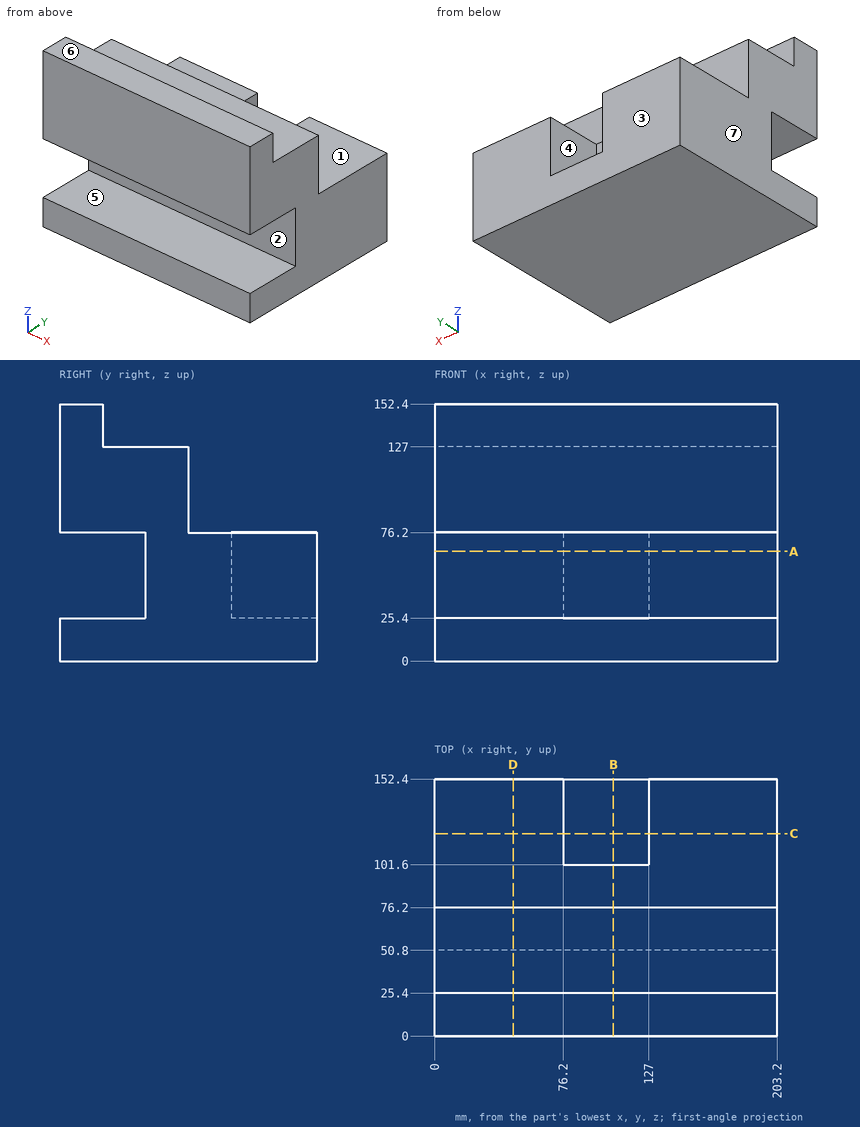
Print and shaded views of the part. All mm, measured from the part's lowest x, y and z. A direction names the side the tool comes from. Round coordinates to 2 decimals unless told otherwise and drop trailing zeros. Loops run counter-clockwise (first coordinate to the right, second up) from the corner with the lowest first, then second, coordinate; pieces in that order, holes last. Notation, with made-up numbers: M -19.75,-5.75 L 9.25,-5.75 A26 ccw 9.25,22.25 Z; hole C 80,26 d8. An arc over 180 degrees is marked long. One line per question, with ' | ' between items.
1) Band-saw the part on A-A (z = 65). Give the cut face in (x, y), then the cut area to 3 significant figures.
Solved:
outline: M 0,50.8 L 203.2,50.8 L 203.2,152.4 L 127,152.4 L 127,101.6 L 76.2,101.6 L 76.2,152.4 L 0,152.4 Z | area: 18,100 mm²
2) Band-saw the part on D-D (x = 46.5). Give the cut face in (y, z).
Solved:
outline: M 0,0 L 152.4,0 L 152.4,76.2 L 76.2,76.2 L 76.2,127 L 25.4,127 L 25.4,152.4 L 0,152.4 L 0,76.2 L 50.8,76.2 L 50.8,25.4 L 0,25.4 Z
3) Band-saw the part on C-C (y = 120). Give the cut face in (x, z).
Solved:
outline: M 0,0 L 203.2,0 L 203.2,76.2 L 127,76.2 L 127,25.4 L 76.2,25.4 L 76.2,76.2 L 0,76.2 Z
4) Band-saw the part on B-B (x = 106). Give the cut face in (y, z).
Solved:
outline: M 0,0 L 152.4,0 L 152.4,25.4 L 101.6,25.4 L 101.6,76.2 L 76.2,76.2 L 76.2,127 L 25.4,127 L 25.4,152.4 L 0,152.4 L 0,76.2 L 50.8,76.2 L 50.8,25.4 L 0,25.4 Z
5) Mould opens along Z. For the marked faces 5, 6 and 7 say: +Z half, -Z half, draft (parallel to the pull), parting line (faces both ways), or undercut.
Solved:
face 5: undercut | face 6: +Z half | face 7: draft
6) Flat gauge pins, fed straight in: pin 1 (3 mm diameter, centred on x = 46.5, z = 103.5, fed in from -Y); pin 2 (7.5 mm diameter, centred on x = 125, z = 133.5, fed in from +Y); pin 3 (1 mm diameter, centred on x = 89, z = 73.5, fed in from +Y); pin 4 (6 mm diameter, centred on x = 80.5, z = 85, fed in from +Y). Where does each tip first touch, or does it go through?
Solved:
pin 1: stops at y = 0 | pin 2: stops at y = 25.4 | pin 3: stops at y = 101.6 | pin 4: stops at y = 76.2
7) 3-axis set-ups, long thin cutter, end or side, ignore diameter. For the marked faces 1, 2, 3 and 4: which of +Z, -Z, +X, -X, +Y, -Y reach the whole face in a straight line?
Solved:
face 1: +Z, +X, -X, +Y | face 2: +X, -X, -Y | face 3: +Z, -Z, +X, -X, +Y | face 4: +Z, +Y
8) Drill centre lines: line 1 along Z through (x, y) = (150.5, 34.5); line 2 along Z through (x, y) = (164.5, 9); line 3 along X through (y, z) = (126.5, 39). Where is each one in solid material? Low to high.
Solved:
line 1: z = 0 to 25.4, 76.2 to 127 | line 2: z = 0 to 25.4, 76.2 to 152.4 | line 3: x = 0 to 76.2, 127 to 203.2
